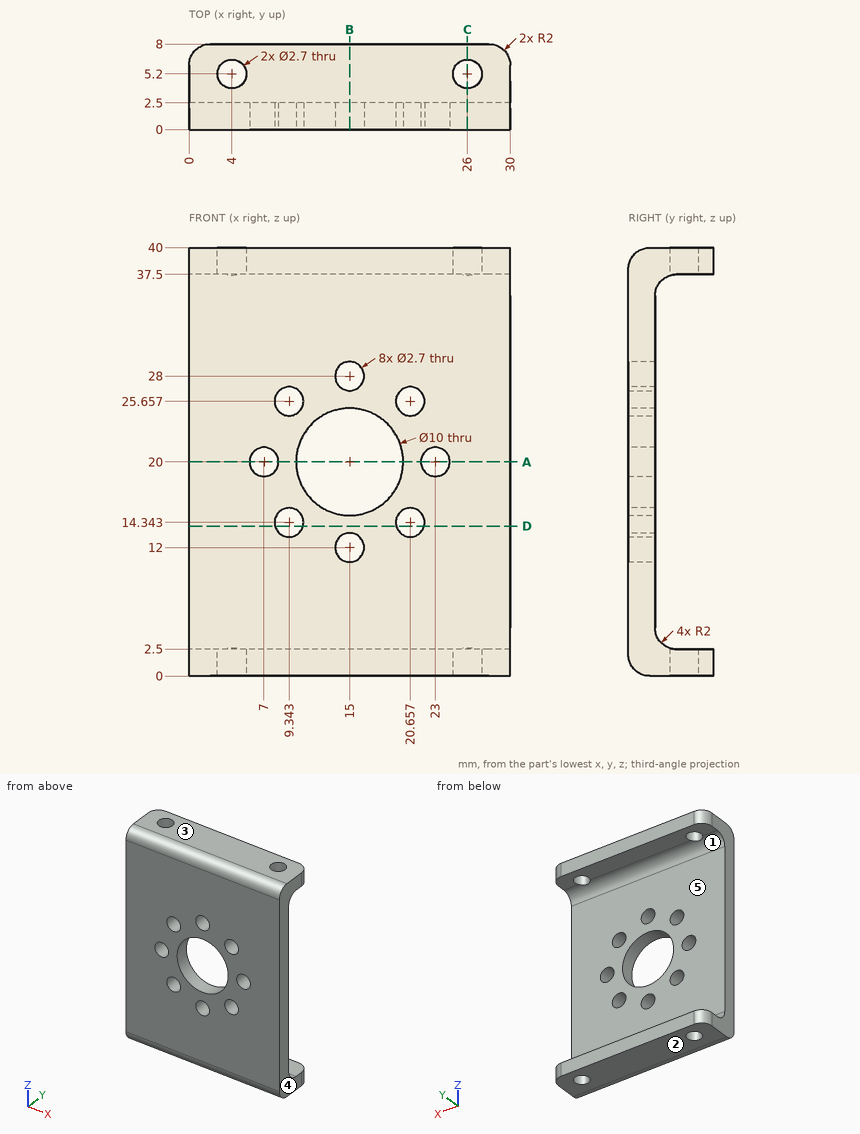
Geometry: see drawing. Coordinates: mm, zero at the bounding-box minimum. A direction names the side the tool comes from. Give positions to 0.01 mm unless a question says otherwise; leave off trailing zeros. Order: outer loops, then holes, each group sorted by start corner. A loop starts at its lowest first (then second) coordinate and runs counter-clockwise, first axis right, second up. Notation, with made-up numbers: (9.25, 31.5) - (14.25, 31.5) arc R15 ccw to (14.25, 54.5) - close; hole circle Ø7 at (45.5, 3). An arc over 180 degrees is marked (long way). Use a Markdown table: item, result.
(1) Line query: line 1 (X direction, y = 5.2, z = 1.6); line 2 (Z direction, x = 8, y = 6.25); line 3 (X direction, y = 2.25, z = 21). Output: solid intervals per line, ascending. Write a range as from..to.
Computed values:
| item | result |
|---|---|
| line 1 | x = 0..2.65, 5.35..24.65, 27.35..30 |
| line 2 | z = 0..2.5, 37.5..40 |
| line 3 | x = 0..6.09, 7.91..10.1, 19.9..22.09, 23.91..30 |
(2) Draft query along Z for the marked faces 3, 4 and 5. Return one class per face: released by +Z, released by -Z, zero draft, split by the parting line, or undercut.
Computed values:
| item | result |
|---|---|
| face 3 | released by +Z |
| face 4 | zero draft |
| face 5 | undercut |
(3) Pin query (flat end, axial travel): pin 1 (9 mm diameter, centred on x = 9.5, z = 23.5, fed in from +Y). Return the tip coordinate at first contact, or that it passes through.
Computed values:
| item | result |
|---|---|
| pin 1 | stops at y = 2.5 |
(4) Access query for the marked faces 1 and 2. Directions: +Z, -Z, +X, -X, +Y, -Y. A direction counts if a zero-diameter tool reaches every point of the face in a straight line with its end or side. Return the directions, or none.
Computed values:
| item | result |
|---|---|
| face 1 | +X, -X, +Y |
| face 2 | -Z, +X, -X, +Y, -Y |
(5) Section query C-C (x = 26). Output: boundary loops of the cut face in (y, z).
Computed values:
| item | result |
|---|---|
| outline | (0, 2) arc R2 ccw to (2, 0) - (3.85, 0) - (3.85, 2.61) arc R2 cw to (2.5, 4.5) - (2.5, 35.5) arc R2 cw to (3.85, 37.39) - (3.85, 40) - (2, 40) arc R2 ccw to (0, 38) - close; (6.55, 0) - (8, 0) - (8, 2.5) - (6.55, 2.5) - close; (6.55, 37.5) - (8, 37.5) - (8, 40) - (6.55, 40) - close |
(6) Section query A-A (z = 20). Output: boundary loops of the cut face in (x, y).
Computed values:
| item | result |
|---|---|
| outline | (0, 0) - (5.65, 0) - (5.65, 2.5) - (0, 2.5) - close; (8.35, 0) - (10, 0) - (10, 2.5) - (8.35, 2.5) - close; (20, 0) - (21.65, 0) - (21.65, 2.5) - (20, 2.5) - close; (24.35, 0) - (30, 0) - (30, 2.5) - (24.35, 2.5) - close |
(7) Section query D-D (z = 14). Output: boundary loops of the cut face in (x, y).
Computed values:
| item | result |
|---|---|
| outline | (0, 0) - (8.04, 0) - (8.04, 2.5) - (0, 2.5) - close; (10.65, 0) - (19.35, 0) - (19.35, 2.5) - (10.65, 2.5) - close; (21.96, 0) - (30, 0) - (30, 2.5) - (21.96, 2.5) - close |
(8) Section query B-B (x = 15). Output: boundary loops of the cut face in (y, z), then the cut area to 3 significant figures.
Computed values:
| item | result |
|---|---|
| outline | (0, 2) arc R2 ccw to (2, 0) - (8, 0) - (8, 2.5) - (4.5, 2.5) arc R2 cw to (2.5, 4.5) - (2.5, 10.65) - (0, 10.65) - close; (0, 13.35) - (2.5, 13.35) - (2.5, 15) - (0, 15) - close; (0, 25) - (2.5, 25) - (2.5, 26.65) - (0, 26.65) - close; (0, 29.35) - (2.5, 29.35) - (2.5, 35.5) arc R2 cw to (4.5, 37.5) - (8, 37.5) - (8, 40) - (2, 40) arc R2 ccw to (0, 38) - close |
| area | 89.0 mm2 |
